Geometry: final body of the model. Coordinates: model frame, mm. Give positions to 0.01 mm unless a question says otherwise; leave off trailing zeros. Write each loop counter-clockwise with the first axis right and the second up, starting at its lowest first coordinate (ties: lowest second). Pieces come first, ordered by that corner, then holes. Notation, with made-up numbers: (-16, -6.5) - (-5, -6.5) arc R14 cw to (-5, 2.5) - close; hole circle Ø9 at (58.5, 19.5). An arc over 180 degrees is marked (long way). Return JSON: item names as keys, results as strings.
from build123d import *

# Parameters (mm, degrees)
F2_DEPTH = 7.30791
F3_DEPTH = 20


with BuildPart() as f2:
    # F0 (on Top) → F2 (new body)
    with BuildSketch(Plane.XY):
        with BuildLine():
            Line((-20, -12.5), (20, -12.5))
            Line((20, -12.5), (20, 12.5))
            Line((20, 12.5), (-20, 12.5))
            ThreePointArc((-20, 12.5), (-11.161165, 8.838835), (-7.5, 0))
            ThreePointArc((-7.5, 0), (-11.161165, -8.838835), (-20, -12.5))
        make_face()
        with BuildLine():
            ThreePointArc((-20, 12.5), (-32.5, 0), (-20, -12.5))
            Line((-20, -12.5), (-20, -5))
            ThreePointArc((-20, -5), (-25, 0), (-20, 5))
            Line((-20, 5), (-20, 12.5))
        make_face()
        with BuildLine():
            Line((-20, -5), (-20, -12.5))
            ThreePointArc((-20, -12.5), (-11.161165, -8.838835), (-7.5, 0))
            ThreePointArc((-7.5, 0), (-11.161165, 8.838835), (-20, 12.5))
            Line((-20, 12.5), (-20, 5))
            ThreePointArc((-20, 5), (-16.464466, 3.535534), (-15, 0))
            ThreePointArc((-15, 0), (-16.464466, -3.535534), (-20, -5))
        make_face()
    extrude(amount=F2_DEPTH)

    # F0 (on Top) → F3 (join)
    with BuildSketch(Plane.XY):
        with BuildLine():
            Line((-20, -5), (-20, -12.5))
            ThreePointArc((-20, -12.5), (-11.161165, -8.838835), (-7.5, 0))
            ThreePointArc((-7.5, 0), (-11.161165, 8.838835), (-20, 12.5))
            Line((-20, 12.5), (-20, 5))
            ThreePointArc((-20, 5), (-16.464466, 3.535534), (-15, 0))
            ThreePointArc((-15, 0), (-16.464466, -3.535534), (-20, -5))
        make_face()
        with BuildLine():
            ThreePointArc((-20, 12.5), (-32.5, 0), (-20, -12.5))
            Line((-20, -12.5), (-20, -5))
            ThreePointArc((-20, -5), (-25, 0), (-20, 5))
            Line((-20, 5), (-20, 12.5))
        make_face()
    extrude(amount=F3_DEPTH)


solid = f2.part
Q1. Section query C-C, the plane x = -11.5. Return the cut outline in (y, z), plus the area to 3 significant figures.
Answer key:
{"outline": "(-12.5, 0) - (12.5, 0) - (12.5, 7.31) - (9.17, 7.31) - (9.17, 20) - (-9.17, 20) - (-9.17, 7.31) - (-12.5, 7.31) - close", "area": "415 mm^2"}
Q2. Material intervals for probe 1 along Y at (x, z) = (-21, 19); probe 2 along Z at (x, y) = (7.5, -3.75); probe 3 along X at (y, z) = (2.75, 3.25), sorted ascending. Write a range as [from, to].
Answer key:
{"probe 1": "y = [-12.46, -4.9], [4.9, 12.46]", "probe 2": "z = [0, 7.31]", "probe 3": "x = [-32.19, -24.18], [-15.82, 20]"}
Q3. Section query B-B, the plane y = 2. Return the cut outline in (x, z).
Answer key:
{"outline": "(-32.34, 0) - (-24.58, 0) - (-24.58, 20) - (-32.34, 20) - close; (-15.42, 0) - (20, 0) - (20, 7.31) - (-7.66, 7.31) - (-7.66, 20) - (-15.42, 20) - close"}
Q4. Section query D-D, the plane x = -6. Return the cut outline in (y, z), plus the area to 3 significant figures.
Answer key:
{"outline": "(-12.5, 0) - (12.5, 0) - (12.5, 7.31) - (-12.5, 7.31) - close", "area": "183 mm^2"}
Q5. Pin query (flat end, axial travel): P1, Ø10, axis at x = 10.5, y = 9.5, coming from the +Z side; P2, Ø2, axis at y = 9, z = 17, coming from the +X side; P3, Ø1, axis at x = -12, z = 15, coming from the +Y side; P4, Ø8, axis at x = -19.5, z = 10, coming from the +Y side. Return the tip coordinate at first contact, or that it passes through.
Answer key:
{"P1": "stops at z = 7.31", "P2": "stops at x = -10.4", "P3": "stops at y = 10", "P4": "stops at y = 12.5"}
Q6. Section query A-A, the plane z = 11. Return the cut outline in (x, y).
Answer key:
{"outline": "(-20, -12.5) arc R12.5 ccw to (-7.5, 0) arc R12.5 ccw (long way) to start; hole circle Ø10 at (-20, 0)"}
